Source: CAD feature listing. Evaluate the final solid. Frame: model axes, mm. A direction names the side the tool comes from. Round coordinates to 2 decimals unless told otherwise and drop trailing zeros. Loops run counter-clockwise (first coordinate to the right, second up) from the corner with the lowest first, then second, coordinate; pieces in that order, holes last.
(1) Section A-A, the plane y = 0. Return the cut outline in (x, z), plus the area to 3 significant figures.
(2) Set-up query: faces 1 (the flat face through (2, -2, -66)), 2 (the flat face through (2, -2, 66)), 3 (the flat face through (0, 0, 70)). Return all of +Z, -Z, +X, -X, +Y, -Y with unobstructed straight access to the full face (end or side cutting, diameter ignored); none if empty.
(3) Material intervals for probe 1 along Z at (x, y) = (3, -1.25); probe 2 along X at (y, z) = (2.25, -21); probe 3 along X at (y, z) = (1.5, -61.5), sorted ascending.
(4) First-contact query: pin 1 Ø3 at (x, z) = (-2.5, -48) entering from -Y; pin 2 Ø1 at (x, z) = (-1, -22) entering from -Y. Flat tips, straight axial feed; report the tip coordinate or a pass-through.
(5) Section C-C, the plane z = 60. Return the cut outline in (x, y), plus the area to 3 significant figures.
```python
from build123d import *

# Parameters (mm, degrees)
F0_R     = 3.5
F1_DEPTH = 70
F2_R     = 3.5
F2_R_2   = 2.5
F3_DEPTH = 4


# Not quite as in the source:
# - a pattern or mirror of a feature is missing from the dataset's text; its kind, count and spacing are read off the source's solid


with BuildPart() as f1:
    # F0 (on Top) → F1 (new body, symmetric)
    with BuildSketch(Plane.XY):
        Circle(F0_R)
    extrude(amount=F1_DEPTH, both=True)

    # F2 (on face) → F3 (cut)
    with BuildSketch(Plane.XY.offset(70)):
        Circle(F2_R)
        Circle(F2_R_2, mode=Mode.SUBTRACT)
    f3 = extrude(amount=-F3_DEPTH, mode=Mode.SUBTRACT)

    # F3_copies: F3 across plane
    add(f3.mirror(Plane(origin=(0, 0, 0), x_dir=(-1, 0, 0), z_dir=(0, 0, -1))), mode=Mode.SUBTRACT)


solid = f1.part
```
Output values:
1. outline: (-3.5, -66) - (-2.5, -66) - (-2.5, -70) - (2.5, -70) - (2.5, -66) - (3.5, -66) - (3.5, 66) - (2.5, 66) - (2.5, 70) - (-2.5, 70) - (-2.5, 66) - (-3.5, 66) - close
1. area: 964 mm2
2. face 1: -Z
2. face 2: +Z
2. face 3: +Z, +X, -X, +Y, -Y
3. probe 1: z = -66 to 66
3. probe 2: x = -2.68 to 2.68
3. probe 3: x = -3.16 to 3.16
4. pin 1: stops at y = -3.35
4. pin 2: stops at y = -3.46
5. outline: circle Ø7 at (0, 0)
5. area: 38.5 mm2
